Autodesk Inventor part; units mm, degrees
ref_plane "YZ Plane" through (0, 0, 0) normal (1, 0, 0) x (0, 1, 0)
ref_plane "XZ Plane" through (0, 0, 0) normal (0, 1, 0) x (-1, 0, 0)
ref_plane "XY Plane" through (0, 0, 0) normal (0, 0, 1) x (1, 0, 0)
sketch "Sketch1" plane through (0, 0, 0) normal (0, 0, 1) x (1, 0, 0)
  line L0 (-17.5, 6.5) -> (17.5, 6.5)
  line L1 (17.5, 6.5) -> (17.5, -6.5)
  line L2 (17.5, -6.5) -> (-17.5, -6.5)
  line L3 (-17.5, -6.5) -> (-17.5, 6.5)
  circle A0 centre (0, 16.5) radius 5
  line L4 (-17.5, 6.5) -> (-3.4801, 20.0901)
  line L5 (17.5, 6.5) -> (3.4801, 20.0901)
  circle A1 centre (0, 16.5) radius 2
  point P0 (0, 0)
  dimension "d0" = 35
  dimension "d1" = 13
  dimension "d5" = 17.5
  dimension "d6" = 6.5
  dimension "d13" = 10
  dimension "d14" = 10
  dimension "d15" = 4
extrude "Extrusion1" add sketch "Sketch1" along normal blind 20 contours L0 L1 L2 L3
extrude "Extrusion3" add sketch "Sketch1" along normal blind 4 contours L4 A0 L5 L0 | A0
mirror "Mirror3" about plane through (0, 0, 0) normal (0, 1, 0) of "Extrusion3"
chamfer "Chamfer1" distance 13 distance2 16 1 edges at (17.5, 0, 20) measured on face at (5.8333, -2.1667, 20)
chamfer "Chamfer2" distance 13 distance2 16 1 edges at (-17.5, 0, 20) measured on face at (-2.8333, -2.1667, 20)
sketch "Sketch2" plane through (-17.5, -6.5, 4) normal (0, -1, 0) x (1, 0, 0)
  line L0 (0, 0) -> (13, 16)
  line L1 (0, 0) -> (35, 0)
  line L2 (22, 16) -> (35, 0)
  line L3 (13, 16) -> (22, 16)
  point P0 (17.5, -4)
  point P1 (17.5, 11)
  dimension "d24" = 35
  dimension "d25" = 17.5
  dimension "d26" = 5
hole "Hole1" at (0, -6.5, 15) direction (0, 1, 0) diameter 2.5 end through all
fillet "Fillet1" radius 5 2 edges at (-4.5, 0, 20) (4.5, 0, 20)
fillet "Fillet2" radius 8 4 edges at (-17.5, -6.5, 2) (-17.5, 6.5, 2) (17.5, -6.5, 2) (17.5, 6.5, 2)
chamfer "Chamfer3" distance 0.8 angle 45 2 edges at (-2, -16.5, 4) (-2, 16.5, 4)
properties part number "3DP_PLA_Part_Detector_Base" material "ABS Plastic"
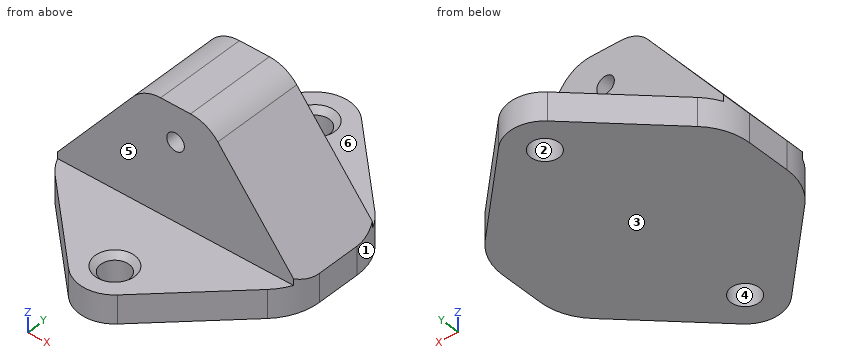
Design review of the part built by this model. Coordinates are the model's own, in mm. Face numbers are marked on the shaded views. A direction names the side the tool comes from. Give positions to 0.01 mm unless a question says otherwise; leave off trailing zeros. Loops run counter-clockwise (first coordinate to the right, second up) from the corner with the lowest first, then second, coordinate; pieces in that order, holes last. Notation, with made-up numbers: M -21,84 L -4,84 A11 cw -4,102 Z; hole C -11,58.5 d5. An arc over 180 degrees is marked long. Write item = value, one per line.
Q1. We need section C-C (y = -16.5). Give the boundary of the cut face in (x, z).
Output values:
outline = M -7.18,0 L -2,0 L -2,3.2 L -2.8,4 L -7.18,4 Z; M 2,0 L 7.18,0 L 7.18,4 L 2.8,4 L 2,3.2 Z
Q2. We need section A-A (x = 0). Give the boundary of the cut face in (y, z), plus the area to 3 significant figures.
Output values:
outline = M -21.5,0 L -18.5,0 L -18.5,3.2 L -19.3,4 L -21.5,4 Z; M -14.5,0 L 14.5,0 L 14.5,3.2 L 13.7,4 L 6.5,4 L 6.5,13.75 L -6.5,13.75 L -6.5,4 L -13.7,4 L -14.5,3.2 Z; M -6.5,16.25 L 6.5,16.25 L 6.5,20 L -6.5,20 Z; M 18.5,0 L 21.5,0 L 21.5,4 L 19.3,4 L 18.5,3.2 Z
area = 314 mm^2
Q3. For the marked faces 4, 5 and 6, list the 3-axis set-ups (+Z, -Z, +X, -X, +Y, -Y) from which the entire face can be reached by the end or side of a thin tool; tool diameter is ignored.
Output values:
face_4 = +Z, -Z
face_5 = +Z, +X, -X, -Y
face_6 = +Z, +X, -X, +Y
Q4. We need section D-D (z = 15). Give the boundary of the cut face in (x, y), plus the area to 3 significant figures.
Output values:
outline = M -8.56,-6.5 L -1.25,-6.5 L -1.25,6.5 L -8.56,6.5 Z; M 1.25,-6.5 L 8.56,-6.5 L 8.56,6.5 L 1.25,6.5 Z
area = 190 mm^2
Q5. Draft analysis for pull direction Y (two halves, no side actions). For the marked faces 1, 2 and 3, state which applies: +Y half, -Y half, draft (parallel to the pull), parting line (faces both ways), or undercut.
Output values:
face_1 = +Y half
face_2 = undercut
face_3 = draft
Q6. We need section B-B (y = 0.5). Give the boundary of the cut face in (x, z), plus the area to 3 significant figures.
Output values:
outline = M -17.5,0 L 17.5,0 L 17.5,4 L 6,18.15 A5 ccw 2.12,20 L -2.12,20 A5 ccw -6,18.15 L -17.5,4 Z; hole C 0,15 d2.5
area = 486 mm^2
Q7. Insertion check: pin 1 (4 mm diameter, centred on x = -3, z = 14.5, fed in from +Y); pin 2 (1 mm diameter, centred on x = 2.5, y = -3, fed in from -Z); pin 3 (3.5 mm diameter, centred on x = 0, y = 16.5, fed in from +Z); pin 4 (5 mm diameter, centred on x = -0.5, z = 16.5, fed in from -Y). Each pin has a flat end and moves straight along its axis. Give the tip position at first contact, or say it passes through.
Output values:
pin_1 = 6.5
pin_2 = 0
pin_3 = through
pin_4 = -6.5
Q8. To check wall thickness, follow line 1 (Y direction, x = 0, z = 1.2); line 2 (Z direction, x = 1.5, y = -13); line 3 (Y direction, x = 2, z = 11.5). State the ranges of each line that lie inside material, in increasing order. Write a range as [from, to].
Output values:
line_1 = [-21.5, -18.5], [-14.5, 14.5], [18.5, 21.5]
line_2 = [0, 4]
line_3 = [-6.5, 6.5]
